Read the model definition and answer for the solid it produces. Units are mm, in the model's axes. Coordinates: 2 decimals unless noted, no trailing zeros. Loops run counter-clockwise (first coordinate to the right, second up) from the corner with the lowest first, then second, coordinate; pieces in that order, holes last. Notation, with made-up numbers: M 87,41.25 L 92,41.25 A21 cw 92,66.25 Z; hole C -1.75,87 d4. An arc over 180 degrees is marked long. One line per item, written item: value. Start each with the question number.
1. The part is cut by section A-A (y = -35). Write down the section's boundary in (x, z).
2. The part is cut by section D-D (y = 340.5). Write down the section's boundary in (x, z).
3. The part is cut by section C-C (z = -7). Write down the section's boundary in (x, y), then the cut area to 3 significant figures.
4. A flat-ended cylindrical pin translates along its axis: pin 1 (1 mm diameter, centred on x = 189.5, y = 57, fed in from -Z). Find the tip coordinate at first contact, or state that the pin passes through.
5. The part is cut by section B-B (x = -221). Write down the section's boundary in (y, z).
6. Determine the mould class of faces 1 (the face through (-4, 6, 2)), 2 (the face through (-4, 5, 0)) for opening direction Y: +Y half, -Y half, draft (parallel to the pull), parting line (faces both ways), or undercut.
7. Consider probe 1 along Y at (x, z) = (-95, -3.5); probe 2 along X at (y, z) = (-211, -9.25); probe 3 along Z at (x, y) = (33, 346). Determine where each line is inside the solid, lowest interval first.
```python
from build123d import *

# Parameters (mm, degrees)
SKETCH_1_W          = 636
SKETCH_1_H          = 786
EXTRUDE_1_DEPTH     = 2
SKETCH_2_W          = 636
SKETCH_2_H          = 786
SKETCH_2_W_2        = 632
SKETCH_2_H_2        = 782
EXTRUDE_2_DEPTH     = 11
SKETCH_3_W          = 636
SKETCH_3_H          = 786
SKETCH_3_W_2        = 616
SKETCH_3_H_2        = 766
EXTRUDE_3_DEPTH     = 2
SKETCH_4_W          = 26
SKETCH_4_H          = 103
CUT_EXTRUDE_1_DEPTH = 10


with BuildPart() as part:
    # 草图1 → 凸台-拉伸1 (new body)
    with BuildSketch(Plane.XY):
        Rectangle(SKETCH_1_W, SKETCH_1_H)
    extrude(amount=EXTRUDE_1_DEPTH)

    # 草图2 → 凸台-拉伸2 (add)
    with BuildSketch(Plane(origin=(0, 0, 0), x_dir=(-1, 0, 0), z_dir=(0, 0, -1))):
        Rectangle(SKETCH_2_W, SKETCH_2_H)
        Rectangle(SKETCH_2_W_2, SKETCH_2_H_2, mode=Mode.SUBTRACT)
    extrude(amount=EXTRUDE_2_DEPTH)

    # 草图3 → 凸台-拉伸3 (add)
    with BuildSketch(Plane(origin=(0, 0, -11), x_dir=(-1, 0, 0), z_dir=(0, 0, -1))):
        Rectangle(SKETCH_3_W, SKETCH_3_H)
        Rectangle(SKETCH_3_W_2, SKETCH_3_H_2, mode=Mode.SUBTRACT)
    extrude(amount=EXTRUDE_3_DEPTH)

    # 草图4 → 切除-拉伸1 (cut)
    with BuildSketch(Plane.XY.offset(2)):
        with Locations((-280, 0)):
            Rectangle(SKETCH_4_W, SKETCH_4_H)
    extrude(amount=-CUT_EXTRUDE_1_DEPTH, mode=Mode.SUBTRACT)


solid = part.part
```
Answer block:
1. outline: M -318,-13 L -308,-13 L -308,-11 L -316,-11 L -316,0 L -293,0 L -293,2 L -318,2 Z; M -267,0 L 316,0 L 316,-11 L 308,-11 L 308,-13 L 318,-13 L 318,2 L -267,2 Z
2. outline: M -318,-13 L -308,-13 L -308,-11 L -316,-11 L -316,0 L 316,0 L 316,-11 L 308,-11 L 308,-13 L 318,-13 L 318,2 L -318,2 Z
3. outline: M -318,-393 L 318,-393 L 318,393 L -318,393 Z; hole M -316,-391 L 316,-391 L 316,391 L -316,391 Z
3. area: 5,670 mm2
4. pin 1: stops at z = 0
5. outline: M -393,-13 L -383,-13 L -383,-11 L -391,-11 L -391,0 L 391,0 L 391,-11 L 383,-11 L 383,-13 L 393,-13 L 393,2 L -393,2 Z
6. face 1: draft
6. face 2: undercut
7. probe 1: y = -393 to -391, 391 to 393
7. probe 2: x = -318 to -316, 316 to 318
7. probe 3: z = 0 to 2
